```python
from build123d import *

# Parameters (mm, degrees)
BOSS_EXTRUDE1_DEPTH = 25.4
SKETCH2_R           = 3.175
CUT_EXTRUDE1_DEPTH  = 25.4
SKETCH3_R           = 3.175
CUT_EXTRUDE2_DEPTH  = 25.4


with BuildPart() as part:
    # Sketch1 → Boss-Extrude1 (new body)
    with BuildSketch(Plane(origin=(0, 0, 0), x_dir=(1, 0, 0), z_dir=(0, 1, 0))):
        Polygon((0, 0), (25.4, 0), (25.4, 25.4), (22.225, 25.4), (22.225, 3.175), (0, 3.175), align=None)
    extrude(amount=BOSS_EXTRUDE1_DEPTH)

    # Sketch2 → Cut-Extrude1 (cut)
    with BuildSketch(Plane(origin=(25.4, 0, 0), x_dir=(0, 0, -1), z_dir=(1, 0, 0))):
        with Locations((12.7, 12.7)):
            Circle(SKETCH2_R)
    extrude(amount=-CUT_EXTRUDE1_DEPTH, mode=Mode.SUBTRACT)

    # Sketch3 → Cut-Extrude2 (cut)
    with BuildSketch(Plane.XY):
        with Locations((12.7, 12.7)):
            Circle(SKETCH3_R)
    extrude(amount=-CUT_EXTRUDE2_DEPTH, mode=Mode.SUBTRACT)


solid = part.part
```
Can you work these out from the model? Positions are in its coordinate system, mm. A direction names the side the tool comes from. Coordinates: 2 decimals unless noted, no trailing zeros. Order: outer loops, then holes, each group sorted by start corner. A loop starts at its lowest first (then second) coordinate and runs counter-clockwise, first axis right, second up.
1. If we section it at B-B (x = 12.7): Please give me the cut outline in (y, z) (3 decimals), then the cut area to 3 significant figures.
2. Thinking about a two-plate mould opening in Y: for faces 3 (the face through (24, 13, -25.4)), 4 (the face through (23.83, 10.77, -10.18)), 5 (the face through (18, 0, -2)), which applies, +Y half, -Y half, draft (parallel to the pull), parting line (faces both ways), or undercut?
3. If we section it at D-D (y = 18.75): Please give me the cut outline in (x, z) (3 decimals).
4. I'm going to push flat-ended pins straight in: pin 1 (1.5 mm diameter, centred on x = 14.5, y = 20, fed in from -Z) (3 decimals); pin 2 (11 mm diameter, centred on y = 9, z = -15, fed in from -X) (3 decimals). Where does each tip first touch, or does it pass through?
5. For faces 1 (the face through (18, 25.4, -2)), 2 (the face through (22.225, 13, -17)), which set-ups out of +Z, -Z, +X, -X, +Y, -Y let a thin tool reach every point of the face, with its end or its side?
6. If we section it at C-C (z = -12.7): Please give me the cut outline in (x, y) (3 decimals), then the cut area to 3 significant figures.
7. If we section it at A-A (y = 12.7): Please give me the cut outline in (x, z) (3 decimals), then the cut area to 3 significant figures.
8. I need wall thicknesses on line 1 (Y direction, x = 23, z = -12.7) (3 decimals); line 2 (X direction, y = 22.75, z = -14) (3 decimals); line 3 (Z direction, x = 18.25, y = 2.5) (3 decimals). Which ranges of each line are inside material? Lowest first, please.
Entries:
1. outline: (0, -3.175) - (9.525, -3.175) - (9.525, 0) - (0, 0) - close; (15.875, -3.175) - (25.4, -3.175) - (25.4, 0) - (15.875, 0) - close
1. area: 60.5 mm2
2. face 3: draft
2. face 4: undercut
2. face 5: -Y half
3. outline: (0, -3.175) - (22.225, -3.175) - (22.225, -25.4) - (25.4, -25.4) - (25.4, 0) - (0, 0) - close
4. pin 1: stops at z = -3.175
4. pin 2: stops at x = 22.225
5. face 1: +Z, -Z, +X, -X, +Y
5. face 2: -Z, -X, +Y, -Y
6. outline: (22.225, 0) - (25.4, 0) - (25.4, 9.525) - (22.225, 9.525) - close; (22.225, 15.875) - (25.4, 15.875) - (25.4, 25.4) - (22.225, 25.4) - close
6. area: 60.5 mm2
7. outline: (0, -3.175) - (9.525, -3.175) - (9.525, 0) - (0, 0) - close; (15.875, -3.175) - (22.225, -3.175) - (22.225, -9.525) - (25.4, -9.525) - (25.4, 0) - (15.875, 0) - close; (22.225, -25.4) - (25.4, -25.4) - (25.4, -15.875) - (22.225, -15.875) - close
7. area: 111 mm2
8. line 1: y = 0 to 9.525, 15.875 to 25.4
8. line 2: x = 22.225 to 25.4
8. line 3: z = -3.175 to 0
